Read the model definition and answer for the solid it produces. Units are mm, in the model's axes. Face numbers are marked on the shaded views. Give positions to 0.01 mm unless a question says otherwise; leave off trailing zeros. Loops run counter-clockwise (first coordinate to the right, second up) from the corner with the lowest first, then second, coordinate; pieces in that order, holes last. Notation, with made-up numbers: (59, 64.25) -> (111, 64.25) arc R10 ccw to (111, 77.25) -> close; hole circle Ø5 at (64.5, -33). An arc over 180 degrees is marked (long way). Write each question's results on one line, items separated by ' | '. Start each with the question number.
Item 1: Determine the mould class of the marked faces 1, 2, 3 and 4 for opening direction Z: +Z half, -Z half, draft (parallel to the pull), parting line (faces both ways), or undercut.
Item 2: Section D-D on x = 10.5 is taken. Write down the section's boundary in (y, z).
Item 3: Section B-B on y = 4 is taken. Write down the section's boundary in (x, z), and give its area (3 significant figures).
Item 4: Section A-A on x = 0 is taken. Write down the section's boundary in (y, z), and give its area (3 significant figures).
Item 5: Find the intervals of material crossed by line 1 (X direction, y = 2.25, z = 4.5); line 2 (X direction, y = 3.25, z = 0); line 3 (Z direction, x = 15.5, y = 8.75), in increasing order.
Item 6: Each of these flat-tipped pins is pushed along its axis until it touches: P1, Ø5, axis at x = -12, y = 9, coming from the +Z side; P2, Ø2, axis at y = 9.5, z = 17, coming from the -X side; P3, Ø5, axis at y = 4.5, z = 8.5, coming from the -X side. Where does it stop, or does it pass through?
Item 7: Section C-C on z = 2 is taken. Write down the section's boundary in (x, y), and give its area (3 significant figures).
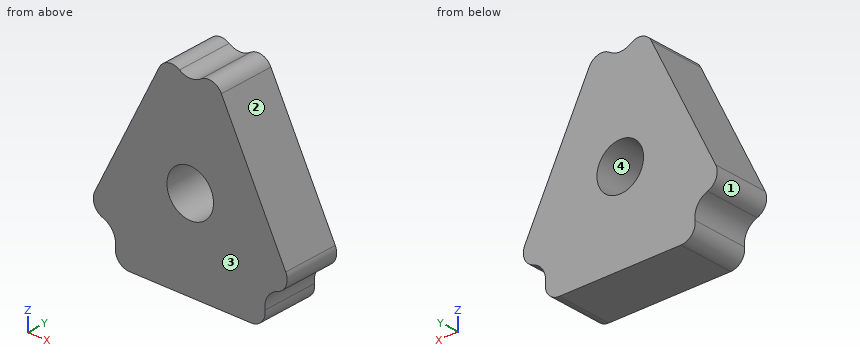
```python
from build123d import *

# Parameters (mm, degrees)
SKETCH1_R           = 5
BOSS_EXTRUDE1_DEPTH = 12


with BuildPart() as part:
    # Sketch1 → Boss-Extrude1 (new body)
    with BuildSketch(Plane(origin=(0, 0, 0), x_dir=(1, 0, 0), z_dir=(0, 1, 0))):
        with BuildLine():
            Line((-20.479322087, 7.014372264), (-6.676095441, -20.592081028))
            ThreePointArc((-6.676095441, -20.592081028), (-4.735248894, -22.157120519), (-2.281607925, -21.714537281))
            ThreePointArc((-2.281607925, -21.714537281), (0, -21), (2.281607925, -21.714537281))
            ThreePointArc((2.281607925, -21.714537281), (4.735248894, -22.157120519), (6.676095441, -20.592081028))
            Line((6.676095441, -20.592081028), (20.479322087, 7.014372264))
            ThreePointArc((20.479322087, 7.014372264), (20.566845751, 9.506073196), (18.740594579, 11.203436029))
            ThreePointArc((18.740594579, 11.203436029), (16.597396767, 12.897075552), (16.041026726, 15.571428571))
            ThreePointArc((16.041026726, 15.571428571), (15.339583608, 17.963961012), (13.07179677, 19))
            Line((13.07179677, 19), (-13.07179677, 19))
            ThreePointArc((-13.07179677, 19), (-15.339583608, 17.963961012), (-16.041026726, 15.571428571))
            ThreePointArc((-16.041026726, 15.571428571), (-16.597396767, 12.897075552), (-18.740594579, 11.203436029))
            ThreePointArc((-18.740594579, 11.203436029), (-20.566845751, 9.506073196), (-20.479322087, 7.014372264))
        make_face()
        with Locations(Location((0, 0, 0), (0, 0, 270))):
            Circle(SKETCH1_R, mode=Mode.SUBTRACT)
    extrude(amount=BOSS_EXTRUDE1_DEPTH)


solid = part.part
```
Findings:
1) face 1: parting line | face 2: +Z half | face 3: draft | face 4: undercut
2) outline: (0, -19) -> (12, -19) -> (12, 12.94) -> (0, 12.94) -> close
3) outline: (-20.48, -7.01) arc R3 ccw to (-18.74, -11.2) arc R4 cw to (-16.04, -15.57) arc R3 ccw to (-13.07, -19) -> (13.07, -19) arc R3 ccw to (16.04, -15.57) arc R4 cw to (18.74, -11.2) arc R3 ccw to (20.48, -7.01) -> (6.68, 20.59) arc R3 ccw to (2.28, 21.71) arc R4 cw to (-2.28, 21.71) arc R3 ccw to (-6.68, 20.59) -> close; hole circle Ø10 at (0, 0) | area: 1,110 mm2
4) outline: (0, -19) -> (12, -19) -> (12, -5) -> (0, -5) -> close; (0, 5) -> (12, 5) -> (12, 21) -> (0, 21) -> close | area: 360 mm2
5) line 1: -14.72 to -2.18, 2.18 to 14.72 | line 2: -16.97 to -5, 5 to 16.97 | line 3: -17.76 to 2.94
6) P1: z = 14.94 | P2: x = -8.97 | P3: x = -13.97
7) outline: (-15.97, 0) -> (-4.58, 0) -> (-4.58, 12) -> (-15.97, 12) -> close; (4.58, 0) -> (15.97, 0) -> (15.97, 12) -> (4.58, 12) -> close | area: 273 mm2
